For this review, take the finished solid that the model builds, in its own axes (mm). Coordinates: 2 decimals unless noted, no trailing zeros. Order: outer loops, then holes, each group sorted by start corner. A loop starts at its lowest first (then second) coordinate and runs counter-clockwise, first axis right, second up. Notation, with made-up numbers: (-8.75, -11.75) - (45.25, -11.75) arc R31 ccw to (45.25, 12.25) - close; hole circle Ø2 at (-26, 84). An arc over 180 degrees is marked (long way). One line per item, written item: value. Start each with the question number.
(1) Clearance check with flat-ended pins moving along their axes: pin 1 (1 mm diameter, centred on x = 13, z = 0.5, fed in from -Y); pin 2 (1 mm diameter, centred on x = -1.5, z = 1, fed in from -Y); pin 3 (1.5 mm diameter, centred on y = 12, z = 1, fed in from -X). State where each tip first meets the part, or that it passes through.
(2) Consider section D-D on y = 26. Write out the cut boundary in (x, z).
(3) Consider section B-B on x = 25.5. Write out the cut boundary in (y, z), then the cut area to 3 significant figures.
(4) Consider section C-C on y = 0. Write out the cut boundary in (x, z), then the cut area to 3 significant figures.
(5) Consider section A-A on z = 2.6. Write out the cut boundary in (x, y) (3 decimals), then the cut area to 3 significant figures.
(6) To check wall thickness, follow line 1 along Y through (x, z) = (7.5, 0.55); line 2 along Y through (x, z) = (19, 1.6); line 3 along X through (y, z) = (87, 1.75). State the ranges of each line that lie inside material, in increasing order.
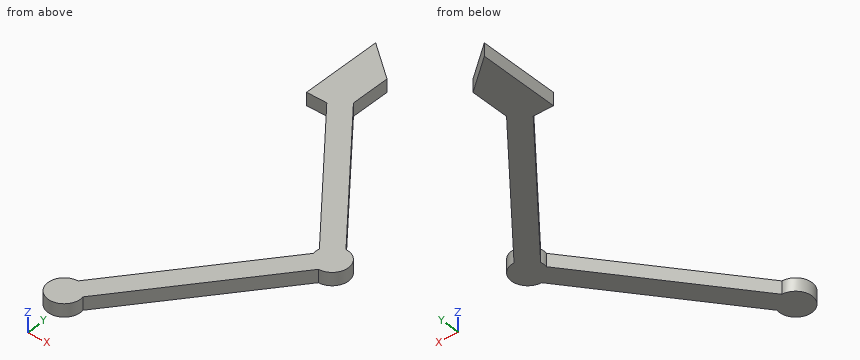
```python
from build123d import *

# Parameters (mm, degrees)
BOSS_EXTRUDE1_DEPTH = 3.18


with BuildPart() as part:
    # Sketch1 → Boss-Extrude1 (new body)
    with BuildSketch(Plane.XY):
        with BuildLine():
            Line((0, 4), (28.125, 39.128113741))
            ThreePointArc((28.125, 39.128113741), (28.028123749, 40.003113741), (28.125, 40.878113741))
            Line((28.125, 40.878113741), (0, 76.006227482))
            Line((0, 76.006227482), (-5, 76.006227482))
            Line((-5, 76.006227482), (-5, 96.006227482))
            Line((-5, 96.006227482), (3.838218952, 88.929989064))
            Line((3.838218952, 88.929989064), (3.838218952, 79.20730223))
            Line((3.838218952, 79.20730223), (3.903123749, 79.131227482))
            Line((3.903123749, 79.131227482), (32.028123749, 44.003113741))
            ThreePointArc((32.028123749, 44.003113741), (36.028123749, 40.003113741), (32.028123749, 36.003113741))
            Line((32.028123749, 36.003113741), (3.903123749, 0.875))
            ThreePointArc((3.903123749, 0.875), (-2.5, -3.122498999), (0, 4))
        make_face()
    extrude(amount=BOSS_EXTRUDE1_DEPTH)


solid = part.part
```
Geometry check:
1. pin 1: stops at y = 11.61
1. pin 2: stops at y = -3.87
1. pin 3: stops at x = 5.8
2. outline: (17.61, 0) - (24.02, 0) - (24.02, 3.18) - (17.61, 3.18) - close
3. outline: (27.85, 0) - (35.85, 0) - (35.85, 3.18) - (27.85, 3.18) - close; (44.16, 0) - (52.16, 0) - (52.16, 3.18) - (44.16, 3.18) - close
3. area: 50.9 mm^2
4. outline: (-4, 0) - (4, 0) - (4, 3.18) - (-4, 3.18) - close
4. area: 25.4 mm^2
5. outline: (-5, 76.006) - (0, 76.006) - (28.125, 40.878) arc R4 ccw to (28.125, 39.128) - (0, 4) arc R4 ccw (long way) to (3.903, 0.875) - (32.028, 36.003) arc R4 ccw to (32.028, 44.003) - (3.903, 79.131) - (3.838, 79.207) - (3.838, 88.93) - (-5, 96.006) - close
5. area: 681 mm^2
6. line 1: y = 5.37 to 13.37, 66.64 to 74.64
6. line 2: y = 19.73 to 27.73, 52.28 to 60.28
6. line 3: x = -5 to 3.84
